For this review, take the finished solid that the model builds, in its own axes (mm). Face numbers are marked on the shaded views. A direction names the side the tool comes from. Give positions to 0.01 mm unless a question says otherwise; leave off trailing zeros. Order: outer loops, then holes, each group sorted by start corner. A loop starts at its lowest first (then second) coordinate and runs counter-clockwise, first axis right, second up. Notation, with made-up numbers: (-35.75, 28.5) - (15.25, 28.5) arc R30 cw to (15.25, 63.5) - close; hole circle Ø5 at (-14, 36.25). An arc over 180 degrees is marked (long way). Answer as a JSON object with one key per item and string values. Group by question number.
from build123d import *

# Parameters (mm, degrees)
SKETCH2_W           = 120
SKETCH2_H           = 90
SKETCH2_W_2         = 87
SKETCH2_H_2         = 70
BOSS_EXTRUDE1_DEPTH = 20
SKETCH3_W           = 7
SKETCH3_H           = 11.2
SKETCH4_R           = 9.5
CUT_EXTRUDE1_DEPTH  = 121
FILLET1_R           = 20
SKETCH5_R           = 5
CUT_EXTRUDE2_DEPTH  = 21


with BuildPart() as part:
    # Sketch2 → Boss-Extrude1 (new body)
    with BuildSketch(Plane(origin=(0, 0, 0), x_dir=(1, 0, 0), z_dir=(0, 1, 0))):
        Rectangle(SKETCH2_W, SKETCH2_H)
        Rectangle(SKETCH2_W_2, SKETCH2_H_2, mode=Mode.SUBTRACT)
    extrude(amount=BOSS_EXTRUDE1_DEPTH)

    # Sketch3 → Cut-Revolve1 (revolve, cut)
    with BuildSketch(Plane(origin=(0, 20, 0), x_dir=(1, 0, 0), z_dir=(0, 1, 0))):
        with Locations((-51.75, 5.6)):
            Rectangle(SKETCH3_W, SKETCH3_H)
        with Locations((51.75, 5.6)):
            Rectangle(SKETCH3_W, SKETCH3_H)
    revolve(axis=Axis((55.25, 20, 0), (-1, 0, 0)), mode=Mode.SUBTRACT)

    # Sketch4 → Cut-Extrude1 (cut, through all)
    with BuildSketch(Plane(origin=(60, 0, 0), x_dir=(0, 0, -1), z_dir=(1, 0, 0))):
        with Locations((0, 20)):
            Circle(SKETCH4_R)
    extrude(amount=-CUT_EXTRUDE1_DEPTH, mode=Mode.SUBTRACT)

    # Fillet1
    fillet1_edges = [part.edges().sort_by_distance(p)[0] for p in [
        (-43.5, 10, -35),
        (-43.5, 10, 35),
        (43.5, 10, 35),
        (43.5, 10, -35),
        (-60, 10, -45),
        (60, 10, -45),
        (60, 10, 45),
        (-60, 10, 45),
    ]]
    fillet(fillet1_edges, radius=FILLET1_R)

    # Sketch5 → Cut-Extrude2 (cut, through all)
    with BuildSketch(Plane(origin=(0, 20, 0), x_dir=(1, 0, 0), z_dir=(0, 1, 0))):
        with Locations((0, -35)):
            Circle(SKETCH5_R)
        with Locations((0, 35)):
            Circle(SKETCH5_R)
    extrude(amount=-CUT_EXTRUDE2_DEPTH, mode=Mode.SUBTRACT)


solid = part.part
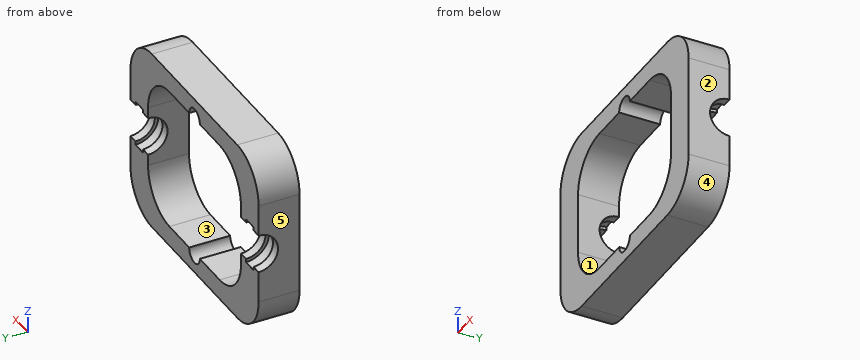
1) Consider section C-C (y = 4.5). Give the boundary of the cut face in (x, z), plus the area to 3 significant figures.
2) For line 1 (X direction, y = 8, z = 11.5); line 2 (Z direction, x = -0.5, y = 15.25); line 3 (Z direction, x = -3, y = 7.5), list the stretches that pass through material, from the lowest coordinate up.
3) Consider section A-A (z = 0). Give the boundary of the cut face in (x, y), plus the area to 3 significant figures.
4) For the marked faces 1 and 2, list the 3-axis set-ups (+Z, -Z, +X, -X, +Y, -Y) from which the entire face can be reached by the end or side of a thin tool; tool diameter is ignored.
5) Mouldability with a two-part tool opening along X and no side actions: class the marked faces 3, 4 and 5 as released by +X, released by -X, zero draft, split by the parting line, or undercut.
6) Consider section D-D (z = 38.5). Give the boundary of the cut face in (x, y), plus the area to 3 significant figures.
7) For pin 1 (8 mm diameter, centred on y = 5, z = 34.5, fed in from -X), flat-tipped, find the tip position at first contact; note if it passes through.
8) Consider section B-B (x = 19.5). Give the boundary of the cut face in (y, z).
Result set:
{
 "1": {"outline": "(-60, -25) arc R20 ccw to (-40, -45) - (40, -45) arc R20 ccw to (60, -25) - (60, 25) arc R20 ccw to (40, 45) - (-40, 45) arc R20 ccw to (-60, 25) - close; hole (-43.5, -15) arc R20 ccw to (-23.5, -35) - (-5, -35) arc R5 ccw to (5, -35) - (23.5, -35) arc R20 ccw to (43.5, -15) - (43.5, 15) arc R20 ccw to (23.5, 35) - (5, 35) arc R5 ccw to (-5, 35) - (-23.5, 35) arc R20 ccw to (-43.5, 15) - close", "area": "4,630 mm2"},
 "2": {"line 1": "x = -60 to -43.5, 43.5 to 60", "line 2": "z = -45 to -39.97, 39.97 to 45", "line 3": "z = -45 to -39, 39 to 45"},
 "3": {"outline": "(-60, 0) - (-43.5, 0) - (-43.5, 10.5) - (-48.25, 10.5) - (-48.25, 8.8) - (-55.25, 8.8) - (-55.25, 10.5) - (-60, 10.5) - close; (43.5, 0) - (60, 0) - (60, 10.5) - (55.25, 10.5) - (55.25, 8.8) - (48.25, 8.8) - (48.25, 10.5) - (43.5, 10.5) - close", "area": "323 mm2"},
 "4": {"face 1": "+Y, -Y", "face 2": "+Z, -Z, +X, +Y, -Y"},
 "5": {"face 3": "undercut", "face 4": "released by +X", "face 5": "released by -X"},
 "6": {"outline": "(-54.76, 0) - (-3.57, 0) - (-3.57, 20) - (-54.76, 20) - close; (3.57, 0) - (54.76, 0) - (54.76, 20) - (3.57, 20) - close", "area": "2,050 mm2"},
 "7": {"pin 1": "stops at x = -59.23"},
 "8": {"outline": "(0, -45) - (20, -45) - (20, -35) - (0, -35) - close; (0, 35) - (20, 35) - (20, 45) - (0, 45) - close"}
}
